Here's how the part is built. I have some questions about the finished solid (model axes, mm). A direction names the side the tool comes from. Coordinates: 2 decimals unless noted, no trailing zeros. Loops run counter-clockwise (first coordinate to the right, second up) from the corner with the lowest first, then second, coordinate; pieces in that order, holes last.
from build123d import *

# Parameters (mm, degrees)
SKETCH1_W            = 130
SKETCH1_H            = 63
BOSS_EXTRUDE1_DEPTH  = 15
LPATTERN1_COUNT      = 2
LPATTERN1_PITCH      = 46.5
LPATTERN1_COUNT_DIR2 = 2
LPATTERN1_PITCH_DIR2 = 46.5
LPATTERN2_COUNT      = 2
LPATTERN2_PITCH      = 100
LPATTERN2_COUNT_DIR2 = 2
LPATTERN2_PITCH_DIR2 = 46.5
SKETCH6_R            = 10
BOSS_EXTRUDE2_DEPTH  = 588
SKETCH7_R            = 10
BOSS_EXTRUDE3_DEPTH  = 588
SKETCH10_W           = 40
SKETCH10_H           = 40
SKETCH10_W_2         = 18
SKETCH10_H_2         = 30
CUT_EXTRUDE1_DEPTH   = 10


with BuildPart() as part:
    # Sketch1 → Boss-Extrude1 (new body)
    with BuildSketch(Plane.XY.offset(89)):
        Rectangle(SKETCH1_W, SKETCH1_H)
    extrude(amount=-BOSS_EXTRUDE1_DEPTH)

    # Sketch2 → Cut-Revolve1 (revolve, cut)
    with BuildSketch(Plane(origin=(23.25, 0, 0), x_dir=(0, 0, -1), z_dir=(1, 0, 0))):
        Polygon((-89, 23.25), (-89, 27.25), (-88.3235, 26.5735), (-74.6765, 26.5735), (-74, 27.25), (-74, 23.25), align=None)
    cut_revolve1 = revolve(axis=Axis((23.25, 23.25, 74), (0, 0, 1)), mode=Mode.SUBTRACT)

    # LPattern1: Cut-Revolve1 2 × 2
    with Locations(*[(-i * LPATTERN1_PITCH, -j * LPATTERN1_PITCH_DIR2, 0) for i in range(LPATTERN1_COUNT) for j in range(LPATTERN1_COUNT_DIR2) if (i, j) != (0, 0)]):
        add(cut_revolve1, mode=Mode.SUBTRACT)

    # Sketch4 → Cut-Revolve2 (revolve, cut)
    with BuildSketch(Plane(origin=(50, 0, 0), x_dir=(0, 0, -1), z_dir=(1, 0, 0))):
        Polygon((-89, 23.25), (-89, 27.75), (-83, 27.75), (-83, 30.75), (-74, 30.75), (-74, 23.25), align=None)
    cut_revolve2 = revolve(axis=Axis((50, 23.25, 74), (0, 0, 1)), mode=Mode.SUBTRACT)

    # LPattern2: Cut-Revolve2 2 × 2
    with Locations(*[(-i * LPATTERN2_PITCH, -j * LPATTERN2_PITCH_DIR2, 0) for i in range(LPATTERN2_COUNT) for j in range(LPATTERN2_COUNT_DIR2) if (i, j) != (0, 0)]):
        add(cut_revolve2, mode=Mode.SUBTRACT)

    # Sketch6 → Boss-Extrude2 (add)
    with BuildSketch(Plane.XY.offset(89)):
        with Locations((-52, 0)):
            Circle(SKETCH6_R)
    extrude(amount=-BOSS_EXTRUDE2_DEPTH)

    # Sketch7 → Boss-Extrude3 (add)
    with BuildSketch(Plane.XY.offset(89)):
        with Locations((52, 0)):
            Circle(SKETCH7_R)
    extrude(amount=-BOSS_EXTRUDE3_DEPTH)

    # Sketch8 → Revolve1 (revolve)
    with BuildSketch(Plane(origin=(0, 0, 0), x_dir=(0, 0, -1), z_dir=(1, 0, 0))):
        Polygon((-74, 0), (-74, 30), (-60.6, 30), (-59, 28.4), (-59, 11), (-50, 11), (-49, 10), (-49, 0), align=None)
    revolve(axis=Axis((0, 0, 49), (0, 0, 1)))

    # Sketch9 → Cut-Revolve3 (revolve, cut)
    with BuildSketch(Plane(origin=(0, 0, 0), x_dir=(0, 0, -1), z_dir=(1, 0, 0))):
        Polygon((-74, 0), (-74, 7.188), (-49.812, 7.188), (-49, 8), (-49, 0), align=None)
    revolve(axis=Axis((0, 0, 49), (0, 0, 1)), mode=Mode.SUBTRACT)

    # Sketch10 → Cut-Extrude1 (cut)
    with BuildSketch(Plane.XY.offset(49)):
        Rectangle(SKETCH10_W, SKETCH10_H)
        Rectangle(SKETCH10_W_2, SKETCH10_H_2, mode=Mode.SUBTRACT)
    extrude(amount=CUT_EXTRUDE1_DEPTH, mode=Mode.SUBTRACT)


solid = part.part
Q1. Suppose I cut it at B-B on x = 0. Write out the boundary of the cut face in (y, z), and give its area (3 significant figures).
Q2. Will these pins go through, and if not, where does the flat tip stop? P1, Ø17, axis at x = -11, y = 9, coming from the -Z side; P2, Ø8, axis at y = 0, z = 52, coming from the +X side; P3, Ø2, axis at x = -7, y = 21, coming from the -Z side; P4, Ø7.5, axis at x = -50.5, y = -23, coming from the -Z side.
Q3. For faces 1 (the flat face through (9, 0, 54)), 2 (the flat face through (65, 0, 82)), 3 (the flat face through (0, 0, 74)), which set-ups out of +Z, -Z, +X, -X, +Y, -Y let a thin tool reach every point of the face, with its end or its side?
Q4. We'd pull the mould along X, two halves only. Please class faces 4 (the flat face through (-1, 31.5, 82)), 5 (the cylindrical face through (57.32, 21.62, 78.44)), 6 (the flat face through (-65, 0, 82)): pulls with the +X half, pulls with the -X half, needs draft (parallel to the pull), parting line crosses it, or undercut.
Q5. Suppose I cut it at A-A on z = -3. Write out the boundary of the cut face in (x, y), and give its area (3 significant figures).
Q6. Please list where these lines run through material, in increasing order: probe 1 along Y at (x, z) = (-23.25, 78); probe 2 along X at (y, z) = (-23, 86); probe 3 along Y at (x, z) = (-50, 85).
Check values:
1. outline: (-31.5, 74) - (-30, 74) - (-30, 60.6) - (-28.4, 59) - (-11, 59) - (-11, 50) - (-10, 49) - (-8, 49) - (-7.19, 49.81) - (-7.19, 74) - (7.19, 74) - (7.19, 49.81) - (8, 49) - (10, 49) - (11, 50) - (11, 59) - (28.4, 59) - (30, 60.6) - (30, 74) - (31.5, 74) - (31.5, 89) - (-31.5, 89) - close
1. area: 1,700 mm2
2. P1: stops at z = 49
2. P2: stops at x = 62
2. P3: stops at z = 59
2. P4: passes through
3. face 1: -Z, +Y, -Y
3. face 2: +Z, -Z, +X, +Y, -Y
3. face 3: -Z
4. face 4: needs draft
4. face 5: undercut
4. face 6: pulls with the -X half
5. outline: circle Ø20 at (-52, 0); circle Ø20 at (52, 0)
5. area: 628 mm2
6. probe 1: y = -31.5 to -26.57, -19.93 to 19.93, 26.57 to 31.5
6. probe 2: x = -65 to -54.49, -45.51 to -26.56, -19.94 to 19.94, 26.56 to 45.51, 54.49 to 65
6. probe 3: y = -31.5 to -27.75, -18.75 to 18.75, 27.75 to 31.5
